from build123d import *

# Parameters (mm, degrees)
F1_DEPTH = 25
F2_R     = 2.5
F3_DEPTH = 25


with BuildPart() as f1:
    # F0 (on Front) → F1 (new body)
    with BuildSketch(Plane.XZ):
        Polygon((6, 5.64185), (0, 5.64185), (0, 0.64185), (5, 0.64185), (5, 3.14185), (6, 3.14185), align=None)
        Polygon((0, 0.64185), (0, 5.64185), (-6, 5.64185), (-6, 3.14185), (-5, 3.14185), (-5, 0.64185), align=None)
    extrude(amount=F1_DEPTH)

    # F2 (on face) → F3 (cut)
    with BuildSketch(Plane.XY.offset(5.64185)):
        with Locations((0, -12.5)):
            Circle(F2_R)
    extrude(amount=-F3_DEPTH, mode=Mode.SUBTRACT)


solid = f1.part
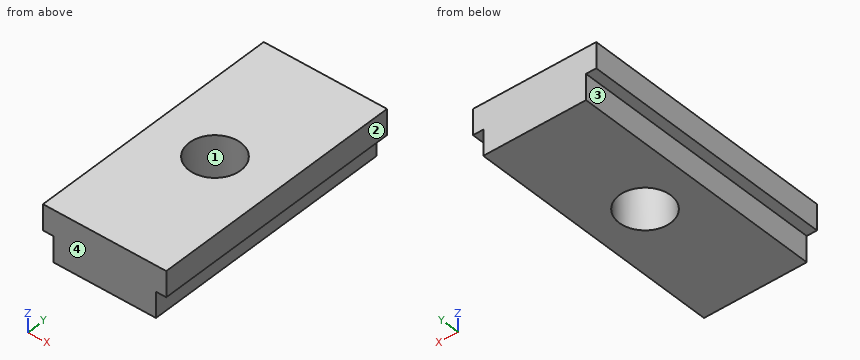
Can you work these out from the model? Positions are in its coordinate system, mm. Face numbers are marked on the shaded views. Give positions to 0.01 mm unless a question says otherwise; leave off trailing zeros. Order: outer loops, then holes, each group sorted by start corner. A loop starts at its lowest first (then second) coordinate and runs counter-clockwise, first axis right, second up. Notation, with made-up numbers: M 77,18.25 L 130,18.25 A16 cw 130,48.25 Z; hole C 59.25,-25 d7. An arc over 180 degrees is marked long. One line per question, with ' | ' between items.
Item 1: Suppose I cut it at A-A, the plane x = 0. Write out the boundary of the cut face in (y, z), then the cut area to 3 significant figures.
Answer block:
outline: M -25,0.64 L -15,0.64 L -15,5.64 L -25,5.64 Z; M -10,0.64 L 0,0.64 L 0,5.64 L -10,5.64 Z | area: 100 mm2
Item 2: We'd pull the mould along X, two halves only. Please class the marked faces 1, 2, 3 and 4: released by +X, released by -X, zero draft, split by the parting line, or undercut.
Answer block:
face 1: undercut | face 2: released by +X | face 3: released by -X | face 4: zero draft
Item 3: Suppose I cut it at B-B, the plane y = -14. Write out the boundary of the cut face in (x, z), then the cut area to 3 significant figures.
Answer block:
outline: M -6,3.14 L -5,3.14 L -5,0.64 L -2,0.64 L -2,5.64 L -6,5.64 Z; M 2,0.64 L 5,0.64 L 5,3.14 L 6,3.14 L 6,5.64 L 2,5.64 Z | area: 35.0 mm2
Item 4: I'm going to push flat-ended pins straight in: pin 1 Ø2 at (y, z) = (-12.5, 2.5) entering from -X; pin 2 Ø0.8 at (y, z) = (-7.5, 1.5) entering from +X. Where does each tip first touch, or does it pass through?
Answer block:
pin 1: stops at x = -6 | pin 2: stops at x = 5
Item 5: Please list where these lines run through material, in increasing order: L1, parallel to Y at x = 0, z = 4.4; L2, parallel to Z at x = -5.5, y = -4; L3, parallel to X at y = -20.5, z = 1.2.
Answer block:
L1: y = -25 to -15, -10 to 0 | L2: z = 3.14 to 5.64 | L3: x = -5 to 5
Item 6: Suppose I cut it at D-D, the plane y = -3. Write out the boundary of the cut face in (x, z).
Answer block:
outline: M -6,3.14 L -5,3.14 L -5,0.64 L 5,0.64 L 5,3.14 L 6,3.14 L 6,5.64 L -6,5.64 Z
Item 7: Suppose I cut it at C-C, the plane z = 2.8. Write out the boundary of the cut face in (x, y), then the cut area to 3 significant figures.
Answer block:
outline: M -5,-25 L 5,-25 L 5,0 L -5,0 Z; hole C 0,-12.5 d5 | area: 230 mm2
